```python
from build123d import *

# Parameters (mm, degrees)
EXTRUDE_1_DEPTH     = 2.7
SKETCH_1_4_W        = 3.35
SKETCH_1_4_H        = 12.4
EXTRUDE_2_DEPTH     = 2
EXTRUDE_START       = 2.7
SKETCH_1_5_W        = 3.35
SKETCH_1_5_H        = 12.4
EXTRUDE_3_DEPTH     = 2
SKETCH_2_R          = 1.75
CUT_EXTRUDE_1_DEPTH = 10.723810981
SKETCH_4_R          = 0.6
CUT_EXTRUDE_2_DEPTH = 9.470684742


with BuildPart() as part:
    # 草图1 → 凸台-拉伸1 (new body)
    with BuildSketch(Plane.XY):
        with BuildLine():
            Line((3.35, 6.2), (0, 6.2))
            Line((0, 6.2), (0, 3.2))
            ThreePointArc((0, 3.2), (2.2627417, 2.2627417), (3.2, 0))
            ThreePointArc((3.2, 0), (2.2627417, -2.2627417), (0, -3.2))
            Line((0, -3.2), (0, -6.2))
            Line((0, -6.2), (3.35, -6.2))
            Line((3.35, -6.2), (3.35, 6.2))
        make_face()
    extrude(amount=EXTRUDE_1_DEPTH)

    # 草图1<4> → 凸台-拉伸2 (add)
    with BuildSketch(Plane.XY):
        with Locations((1.675, 0)):
            Rectangle(SKETCH_1_4_W, SKETCH_1_4_H)
    extrude(amount=-EXTRUDE_2_DEPTH)

    # 草图1<5> → 凸台-拉伸3 (add)
    with BuildSketch(Plane.XY.offset(EXTRUDE_START)):
        with Locations((1.675, 0)):
            Rectangle(SKETCH_1_5_W, SKETCH_1_5_H)
    extrude(amount=EXTRUDE_3_DEPTH)

    # 草图2 → 切除-拉伸1 (cut, through all)
    with BuildSketch(Plane.XY.offset(4.7)):
        Circle(SKETCH_2_R)
    extrude(amount=-CUT_EXTRUDE_1_DEPTH, mode=Mode.SUBTRACT)

    # 草图4 → 切除-拉伸2 (cut, through all)
    with BuildSketch(Plane(origin=(3.35, 0, 0), x_dir=(0, 0, -1), z_dir=(1, 0, 0))):
        with Locations((-1.35, -4.7)):
            Circle(SKETCH_4_R)
        with Locations((-1.35, 4.7)):
            Circle(SKETCH_4_R)
    extrude(amount=-CUT_EXTRUDE_2_DEPTH, mode=Mode.SUBTRACT)


solid = part.part
```
Can you work these out from the model? Positions are in its coordinate system, mm. A direction names the side the tool comes from. Round coordinates to 2 decimals unless told otherwise and drop trailing zeros. Order: outer loops, then holes, each group sorted by start corner. A loop starts at its lowest first (then second) coordinate and runs counter-clockwise, first axis right, second up.
(1) If we section it at A-A (y = -4.7): Please give me the cut outline in (x, z), plus the area to 3 significant figures.
Results are:
outline: (0, -2) - (3.35, -2) - (3.35, 0.75) - (0, 0.75) - close; (0, 1.95) - (3.35, 1.95) - (3.35, 4.7) - (0, 4.7) - close
area: 18.4 mm2
(2) If I drill on L1, parallel to Z at x = 1.3, y = -2; L2, parallel to Y at x = 1.4, z = 1.35; L3, parallel to Y at x = 1.9, z = 1.35, over which ranges is the centre line in solid material (lowest first)?
Results are:
L1: z = -2 to 0, 2.7 to 4.7
L2: y = -6.2 to -5.3, -4.1 to -2.88, 2.88 to 4.1, 5.3 to 6.2
L3: y = -6.2 to -5.3, -4.1 to -2.57, 2.57 to 4.1, 5.3 to 6.2
(3) We'd pull the mould along Y, two halves only. Please class faces 1 (the face through (2, 0, 4.7)), 2 (the face through (2, -6.2, 1)), 3 (the face through (1.75, -0.04, -0.99)), 4 (the face through (2, 0, 2.7)): +Y half, -Y half, draft (parallel to the pull), parting line (faces both ways), or undercut.
Results are:
face 1: draft
face 2: -Y half
face 3: undercut
face 4: undercut
(4) If we section it at C-C (z = 1): Please give me the cut outline in (x, y).
Results are:
outline: (0, -6.2) - (3.35, -6.2) - (3.35, -5.19) - (0, -5.19) - close; (0, -4.21) - (3.35, -4.21) - (3.35, 4.21) - (0, 4.21) - (0, 3.2) arc R3.2 cw to (0, -3.2) - close; (0, 5.19) - (3.35, 5.19) - (3.35, 6.2) - (0, 6.2) - close
(5) If we section it at B-B (x = 0.9): Please give me the cut outline in (y, z), plus the area to 3 significant figures.
Results are:
outline: (-6.2, -2) - (-1.5, -2) - (-1.5, 0) - (-3.07, 0) - (-3.07, 2.7) - (-1.5, 2.7) - (-1.5, 4.7) - (-6.2, 4.7) - close; (1.5, -2) - (6.2, -2) - (6.2, 4.7) - (1.5, 4.7) - (1.5, 2.7) - (3.07, 2.7) - (3.07, 0) - (1.5, 0) - close; hole circle Ø1.2 at (-4.7, 1.35); hole circle Ø1.2 at (4.7, 1.35)
area: 52.2 mm2
(6) If we section it at D-D (x = 3.05): Please give me the cut outline in (y, z).
Results are:
outline: (-6.2, -2) - (6.2, -2) - (6.2, 4.7) - (-6.2, 4.7) - close; hole circle Ø1.2 at (-4.7, 1.35); hole (-0.97, 0) - (0.97, 0) - (0.97, 2.7) - (-0.97, 2.7) - close; hole circle Ø1.2 at (4.7, 1.35)
(7) On a 3-axis mill with a long thin cutter (end or side, diameter ignored), from which of +Z, -Z, +X, -X, +Y, -Y can I reach the whole of each face in a straight line? I mean faces 5 (the face through (2, 0, -2)), 6 (the face through (2, 0, 0)). Say none if no direction works.
Results are:
face 5: -Z, +X, -X, +Y, -Y
face 6: -X
